from build123d import *

# Parameters (mm, degrees)
F1_DEPTH = 7.62


# Not quite as in the source:
# - a feature names something its author has since deleted; it is built from what else it names


with BuildPart() as f1:
    # F0 (on Front) → F1 (new body)
    with BuildSketch(Plane.XZ):
        with BuildLine():
            ThreePointArc((10.3407477596, 18.5977799931), (17.6059784875, 5.3059692522), (20.1200594207, -9.6317416622))
            ThreePointArc((20.1200594207, -9.6317416622), (18.9331000604, -19.9720923089), (15.4339684141, -29.7745308699))
            Line((15.4339684141, -29.7745308699), (15.4339684141, -39.0992002321))
            ThreePointArc((15.4339684141, -39.0992002321), (22.5007653243, -25.1123260967), (24.9346453986, -9.6317416622))
            ThreePointArc((24.9346453986, -9.6317416622), (-40.9946586007, 38.3830978282), (-66.4621167465, -39.0992002321))
            Line((-66.4621167465, -39.0992002321), (-66.4621167465, -29.7745308699))
            ThreePointArc((-66.4621167465, -29.7745308699), (-70.8175510234, -4.1482087801), (-60.473849015, 19.6989298396))
            ThreePointArc((-60.473849015, 19.6989298396), (-58.8829140283, 21.49693763), (-57.1996202187, 23.2087869508))
            ThreePointArc((-57.1996202187, 23.2087869508), (-42.5995223376, 32.6832865075), (-25.5140741662, 36.0023919246))
            ThreePointArc((-25.5140741662, 36.0023919246), (-23.1888304756, 35.9431131373), (-20.869627773, 35.7654307819))
            ThreePointArc((-20.869627773, 35.7654307819), (-6.1592475305, 31.6945796612), (6.3859014459, 23.0005384324))
            ThreePointArc((6.3859014459, 23.0005384324), (8.4347729102, 20.8633387673), (10.3407477596, 18.5977799931))
        make_face()
        with BuildLine():
            Line((15.4339684141, -39.0992002321), (15.4339684141, -29.7745308699))
            ThreePointArc((15.4339684141, -29.7745308699), (12.7227075108, -34.5400269346), (9.459491795, -38.9459674269))
            ThreePointArc((9.459491795, -38.9459674269), (7.971092144, -40.635254131), (6.4011850797, -42.2490741021))
            ThreePointArc((6.4011850797, -42.2490741021), (-6.064908215, -50.9137485421), (-20.6835588609, -55.0094924892))
            ThreePointArc((-20.6835588609, -55.0094924892), (-25.4205342826, -55.265779381), (-30.1585205594, -55.0289141064))
            ThreePointArc((-30.1585205594, -55.0289141064), (-44.8689008019, -50.9580629857), (-57.4140497783, -42.2640217569))
            ThreePointArc((-57.4140497783, -42.2640217569), (-59.4700632753, -40.1188693041), (-61.3821167465, -37.8444634324))
            ThreePointArc((-61.3821167465, -37.8444634324), (-64.1334823406, -33.9425512021), (-66.4621167465, -29.7745308699))
            Line((-66.4621167465, -29.7745308699), (-66.4621167465, -39.0992002321))
            ThreePointArc((-66.4621167465, -39.0992002321), (-25.5140741662, -60.0804612271), (15.4339684141, -39.0992002321))
        make_face()
        with BuildLine():
            Line((15.4339684141, -55.2114608665), (15.4339684141, -39.0992002321))
            ThreePointArc((15.4339684141, -39.0992002321), (-25.5140741662, -60.0804612271), (-66.4621167465, -39.0992002321))
            Line((-66.4621167465, -39.0992002321), (-66.4621167465, -58.9845308699))
            Line((-66.4621167465, -58.9845308699), (-66.4621167465, -67.8745308699))
            Line((-66.4621167465, -67.8745308699), (15.4339684141, -67.8745308699))
            Line((15.4339684141, -67.8745308699), (15.4339684141, -58.9845308699))
            Line((15.4339684141, -58.9845308699), (15.4339684141, -55.2114608665))
        make_face()
        with BuildLine():
            Line((-30.119077868, -4.8424361606), (-57.1996202187, 23.2087869508))
            ThreePointArc((-57.1996202187, 23.2087869508), (-58.8829140283, 21.49693763), (-60.473849015, 19.6989298396))
            Line((-60.473849015, 19.6989298396), (-32.1581321342, -9.6317416622))
            ThreePointArc((-32.1581321342, -9.6317416622), (-31.6271510436, -7.0290896739), (-30.119077868, -4.8424361606))
        make_face()
        with BuildLine():
            Line((-57.4140497783, -42.2640217569), (-30.1585205594, -14.3828072251))
            ThreePointArc((-30.1585205594, -14.3828072251), (-31.6378588353, -12.2090983718), (-32.1581321342, -9.6317416622))
            Line((-32.1581321342, -9.6317416622), (-61.3821167465, -37.8444634324))
            ThreePointArc((-61.3821167465, -37.8444634324), (-59.4700632753, -40.1188693041), (-57.4140497783, -42.2640217569))
        make_face()
        with BuildLine():
            Line((-20.6835588609, -55.0094924892), (-20.6835588609, -14.1934987981))
            ThreePointArc((-20.6835588609, -14.1934987981), (-25.3813532931, -16.2744738901), (-30.1585205594, -14.3828072251))
            Line((-30.1585205594, -14.3828072251), (-30.1585205594, -55.0289141064))
            ThreePointArc((-30.1585205594, -55.0289141064), (-25.4205342826, -55.265779381), (-20.6835588609, -55.0094924892))
        make_face()
        with BuildLine():
            Line((-18.8700161982, -9.6317416622), (10.3407477596, 18.5977799931))
            ThreePointArc((10.3407477596, 18.5977799931), (8.4347729102, 20.8633387673), (6.3859014459, 23.0005384324))
            Line((6.3859014459, 23.0005384324), (-20.869627773, -4.8806760994))
            ThreePointArc((-20.869627773, -4.8806760994), (-19.3902894971, -7.0543849527), (-18.8700161982, -9.6317416622))
        make_face()
        with BuildLine():
            Line((-20.869627773, -4.8806760994), (-20.869627773, 35.7654307819))
            ThreePointArc((-20.869627773, 35.7654307819), (-23.1888304756, 35.9431131373), (-25.5140741662, 36.0023919246))
            Line((-25.5140741662, 36.0023919246), (-25.5140741662, -2.9876836943))
            ThreePointArc((-25.5140741662, -2.9876836943), (-23.006370907, -3.4791055894), (-20.869627773, -4.8806760994))
        make_face()
        with BuildLine():
            ThreePointArc((-20.6835588609, -14.1934987981), (-19.340026467, -12.0862561334), (-18.8700161982, -9.6317416622))
            ThreePointArc((-18.8700161982, -9.6317416622), (-19.3902894971, -7.0543849527), (-20.869627773, -4.8806760994))
            ThreePointArc((-20.869627773, -4.8806760994), (-23.006370907, -3.4791055894), (-25.5140741662, -2.9876836943))
            ThreePointArc((-25.5140741662, -2.9876836943), (-27.9963194101, -3.4687906783), (-30.119077868, -4.8424361606))
            ThreePointArc((-30.119077868, -4.8424361606), (-31.6271510436, -7.0290896739), (-32.1581321342, -9.6317416622))
            ThreePointArc((-32.1581321342, -9.6317416622), (-31.6378588353, -12.2090983718), (-30.1585205594, -14.3828072251))
            ThreePointArc((-30.1585205594, -14.3828072251), (-25.3813532931, -16.2744738901), (-20.6835588609, -14.1934987981))
        make_face()
        with BuildLine():
            Line((9.459491795, -38.9459674269), (-18.8700161982, -9.6317416622))
            ThreePointArc((-18.8700161982, -9.6317416622), (-19.340026467, -12.0862561334), (-20.6835588609, -14.1934987981))
            Line((-20.6835588609, -14.1934987981), (6.4011850797, -42.2490741021))
            ThreePointArc((6.4011850797, -42.2490741021), (7.971092144, -40.635254131), (9.459491795, -38.9459674269))
        make_face()
    extrude(amount=F1_DEPTH)


solid = f1.part
Geometry check sheet. Reference: the model listing, model coordinates, mm. A direction names the side the tool comes from. Give positions to 0.01 mm unless a question says otherwise; leave off trailing zeros. Write each loop counter-clockwise with the first axis right and the second up, starting at its lowest first coordinate (ties: lowest second). Pieces come first, ordered by that corner, then holes.
1) Cross-section at C-C (z = 29.5). Record the boundary of the cut face in (x, y).
Values follow:
outline: (-57.35, -7.62) - (-48.99, -7.62) - (-48.99, 0) - (-57.35, 0) - close; (-25.51, -7.62) - (-20.87, -7.62) - (-20.87, 0) - (-25.51, 0) - close; (-2.04, -7.62) - (6.33, -7.62) - (6.33, 0) - (-2.04, 0) - close
2) Go/stop test with a flat-tipped pin: pin 1 Ø2.5 at (y, z) = (-4, -47.5) entering from -X. Record where the tip stops, or that it passes through.
Values follow:
pin 1: stops at x = -66.46
3) Set-up check for faces 1 (the face through (15.434, -4, -54)), 2 (the face through (-4.469, -3.757, 4.285)), 3 (the face through (-66.462, -4, -53)): record each of +Z, -Z, +X, -X, +Y, -Y from which the full face is reachable in a straight line by a thin tool's end or side.
Values follow:
face 1: -Z, +X, +Y, -Y
face 2: +Y, -Y
face 3: -Z, -X, +Y, -Y
4) Thickness scan on line 1 (X direction, y = -6.5, z = 7.5); line 2 (Z direction, x = -50, y = -6); line 3 (X direction, y = -2.5, z = -36). Record the ranges inside material, lowest first.
Values follow:
line 1: x = -72.96 to -67.81, -48.7 to -42.03, -25.51 to -20.87, -8.77 to -1.14, 16.78 to 21.94
line 2: z = -67.87 to -48.14, -34.68 to -26.86, 8.85 to 15.75, 28.88 to 34.48
line 3: x = -68.52 to -62.76, -59.47 to -51.29, -30.16 to -20.68, 0.37 to 6.61, 11.73 to 17.5
5) Cross-section at B-B (y = -3.5). Record the boundary of the cut face in (x, z), plus the area to 3 significant figures.
Values follow:
outline: (-66.46, -67.87) - (15.43, -67.87) - (15.43, -39.1) arc R50.45 ccw (long way) to (-66.46, -39.1) - close; hole (-61.38, -37.84) - (-32.16, -9.63) - (-60.47, 19.7) arc R45.63 ccw to start; hole (-57.41, -42.26) arc R45.63 ccw to (-30.16, -55.03) - (-30.16, -14.38) - close; hole (-57.2, 23.21) - (-30.12, -4.84) arc R6.64 cw to (-25.51, -2.99) - (-25.51, 36) arc R45.63 ccw to start; hole (-20.87, -4.88) - (6.39, 23) arc R45.63 ccw to (-20.87, 35.77) - close; hole (-20.68, -55.01) arc R45.63 ccw to (6.4, -42.25) - (-20.68, -14.19) - close; hole (-18.87, -9.63) - (9.46, -38.95) arc R45.63 ccw to (10.34, 18.6) - close
area: 4,090 mm2
6) Release check for a two-part mould opening along Z. For faces 4 (the face through (-26, -4, -67.875)), 5 (the face through (-20.87, -4, 15)), 6 (the face through (-26, 0, -25)) record: released by +Z, released by -Z, zero draft, split by the parting line, or undercut.
Values follow:
face 4: released by -Z
face 5: undercut
face 6: zero draft
7) Cross-section at D-D (x = -11). Record the boundary of the cut face in (y, z).
Values follow:
outline: (-7.62, -67.87) - (0, -67.87) - (0, -52.9) - (-7.62, -52.9) - close; (-7.62, -24.22) - (0, -24.22) - (0, -17.78) - (-7.62, -17.78) - close; (-7.62, -2.03) - (0, -2.03) - (0, 5.22) - (-7.62, 5.22) - close; (-7.62, 33.63) - (0, 33.63) - (0, 38.68) - (-7.62, 38.68) - close
8) Cross-section at A-A (x = 8). Record the boundary of the cut face in (y, z), plus the area to 3 significant figures.
Values follow:
outline: (-7.62, -67.87) - (0, -67.87) - (0, -37.44) - (-7.62, -37.44) - close; (-7.62, 16.34) - (0, 16.34) - (0, 28.08) - (-7.62, 28.08) - close
area: 321 mm2
